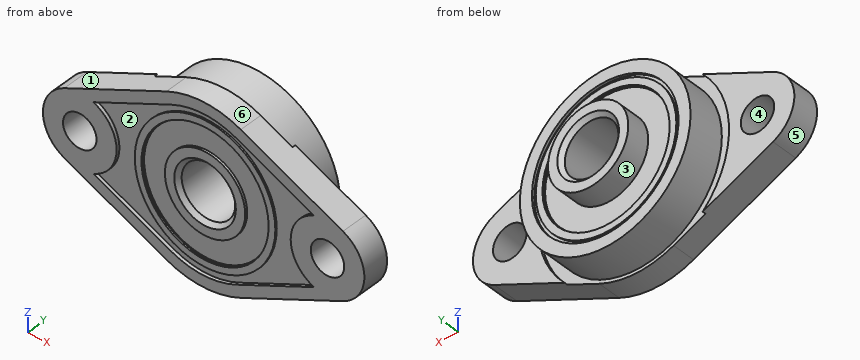
```python
from build123d import *

# Parameters (mm, degrees)
SKETCH2_R               = 2.5
BOSS_EXTRUDE1_DEPTH     = 4
SKETCH3_R               = 14.25
CUT_EXTRUDE1_DEPTH      = 0.5
SKETCH4_R               = 12.75
BOSS_EXTRUDE2_DEPTH     = 5.5
CUT_EXTRUDE2_DEPTH      = 0.5
SKETCH6_R               = 10.95
CUT_EXTRUDE3_DEPTH      = 0.4
SKETCH7_R               = 10.5
BOSS_EXTRUDE3_DEPTH     = 0.25
SKETCH8_R               = 9.5
CUT_EXTRUDE4_DEPTH      = 0.35
SKETCH9_R               = 10.5
BOSS_EXTRUDE4_DEPTH     = 0.25
SKETCH10_R              = 9.5
CUT_EXTRUDE5_DEPTH      = 0.35
SKETCH11_R              = 6
BOSS_EXTRUDE5_DEPTH     = 0.35
SKETCH12_R              = 6
BOSS_EXTRUDE6_DEPTH     = 3.5
SKETCH13_R              = 4
CUT_EXTRUDE6_DEPTH      = 1
CUT_EXTRUDE6_DEPTH_BACK = 13
CHAMFER1_SIZE           = 0.6
CHAMFER2_SIZE           = 0.6
CHAMFER3_SIZE           = 0.1


with BuildPart() as part:
    # Sketch2 → Boss-Extrude1 (new body)
    with BuildSketch(Plane(origin=(0, 0, 0), x_dir=(1, 0, 0), z_dir=(0, 1, 0))):
        with BuildLine():
            Line((-5.550675676, 12.031313293), (-20.804054054, 4.994130046))
            ThreePointArc((-20.804054054, 4.994130046), (-24, 0), (-20.804054054, -4.994130046))
            Line((-20.804054054, -4.994130046), (-5.550675676, -12.031313293))
            ThreePointArc((-5.550675676, -12.031313293), (0, -13.25), (5.550675676, -12.031313293))
            Line((5.550675676, -12.031313293), (20.804054054, -4.994130046))
            ThreePointArc((20.804054054, -4.994130046), (24, 0), (20.804054054, 4.994130046))
            Line((20.804054054, 4.994130046), (5.550675676, 12.031313293))
            ThreePointArc((5.550675676, 12.031313293), (0, 13.25), (-5.550675676, 12.031313293))
        make_face()
        with Locations((-18.5, 0)):
            Circle(SKETCH2_R, mode=Mode.SUBTRACT)
        with Locations((18.5, 0)):
            Circle(SKETCH2_R, mode=Mode.SUBTRACT)
    extrude(amount=BOSS_EXTRUDE1_DEPTH)

    # Sketch3 → Cut-Extrude1 (cut)
    with BuildSketch(Plane(origin=(0, 4, 0), x_dir=(1, 0, 0), z_dir=(0, 1, 0))):
        Circle(SKETCH3_R)
    extrude(amount=-CUT_EXTRUDE1_DEPTH, mode=Mode.SUBTRACT)

    # Sketch4 → Boss-Extrude2 (add)
    with BuildSketch(Plane(origin=(0, 3.5, 0), x_dir=(1, 0, 0), z_dir=(0, 1, 0))):
        Circle(SKETCH4_R)
    extrude(amount=BOSS_EXTRUDE2_DEPTH)

    # Sketch5 → Cut-Extrude2 (cut)
    with BuildSketch(Plane.XZ):
        with BuildLine():
            Line((4.838513514, -10.487673097), (16.48142728, -5.116186488))
            ThreePointArc((16.48142728, -5.116186488), (13, 0), (16.48142728, 5.116186488))
            Line((16.48142728, 5.116186488), (4.838513514, 10.487673097))
            ThreePointArc((4.838513514, 10.487673097), (0, 11.55), (-4.838513514, 10.487673097))
            Line((-4.838513514, 10.487673097), (-16.48142728, 5.116186488))
            ThreePointArc((-16.48142728, 5.116186488), (-13, 0), (-16.48142728, -5.116186488))
            Line((-16.48142728, -5.116186488), (-4.838513514, -10.487673097))
            ThreePointArc((-4.838513514, -10.487673097), (0, -11.55), (4.838513514, -10.487673097))
        make_face()
    extrude(amount=-CUT_EXTRUDE2_DEPTH, mode=Mode.SUBTRACT)

    # Sketch6 → Cut-Extrude3 (cut)
    with BuildSketch(Plane(origin=(0, 9, 0), x_dir=(1, 0, 0), z_dir=(0, 1, 0))):
        Circle(SKETCH6_R)
    extrude(amount=-CUT_EXTRUDE3_DEPTH, mode=Mode.SUBTRACT)

    # Sketch7 → Boss-Extrude3 (add)
    with BuildSketch(Plane(origin=(0, 8.6, 0), x_dir=(1, 0, 0), z_dir=(0, 1, 0))):
        Circle(SKETCH7_R)
    extrude(amount=BOSS_EXTRUDE3_DEPTH)

    # Sketch8 → Cut-Extrude4 (cut)
    with BuildSketch(Plane(origin=(0, 8.85, 0), x_dir=(1, 0, 0), z_dir=(0, 1, 0))):
        Circle(SKETCH8_R)
    extrude(amount=-CUT_EXTRUDE4_DEPTH, mode=Mode.SUBTRACT)

    # Sketch9 → Boss-Extrude4 (add)
    with BuildSketch(Plane.XZ.offset(-0.5)):
        Circle(SKETCH9_R)
    extrude(amount=BOSS_EXTRUDE4_DEPTH)

    # Sketch10 → Cut-Extrude5 (cut)
    with BuildSketch(Plane.XZ.offset(-0.25)):
        Circle(SKETCH10_R)
    extrude(amount=-CUT_EXTRUDE5_DEPTH, mode=Mode.SUBTRACT)

    # Sketch11 → Boss-Extrude5 (add)
    with BuildSketch(Plane.XZ.offset(-0.6)):
        Circle(SKETCH11_R)
    extrude(amount=BOSS_EXTRUDE5_DEPTH)

    # Sketch12 → Boss-Extrude6 (add)
    with BuildSketch(Plane(origin=(0, 8.5, 0), x_dir=(1, 0, 0), z_dir=(0, 1, 0))):
        Circle(SKETCH12_R)
    extrude(amount=BOSS_EXTRUDE6_DEPTH)

    # Sketch13 → Cut-Extrude6 (cut, two sides)
    with BuildSketch(Plane(origin=(0, 12, 0), x_dir=(1, 0, 0), z_dir=(0, 1, 0))) as cut_extrude6_sk:
        Circle(SKETCH13_R)
    extrude(amount=CUT_EXTRUDE6_DEPTH, mode=Mode.SUBTRACT)
    extrude(cut_extrude6_sk.sketch, amount=-CUT_EXTRUDE6_DEPTH_BACK, mode=Mode.SUBTRACT)

    # Chamfer1
    chamfer1_edges = [part.edges().sort_by_distance(p)[0] for p in [
        (-4, 12, 0),
    ]]
    chamfer(chamfer1_edges, length=CHAMFER1_SIZE)

    # Chamfer2
    chamfer2_edges = [part.edges().sort_by_distance(p)[0] for p in [
        (-4, 0.25, 0),
    ]]
    chamfer(chamfer2_edges, length=CHAMFER2_SIZE)

    # Chamfer3
    chamfer3_edges = [part.edges().sort_by_distance(p)[0] for p in [
        (-9.5, 0.6, 0),
        (-9.5, 8.5, 0),
    ]]
    chamfer(chamfer3_edges, length=CHAMFER3_SIZE)


solid = part.part
```
Read the model definition and answer for the solid it produces. Units are mm, in the model's axes. Face numbers are marked on the shaded views. A direction names the side the tool comes from. Give positions to 0.01 mm unless a question says otherwise; leave off trailing zeros. Write each loop counter-clockwise with the first axis right and the second up, starting at its lowest first coordinate (ties: lowest second). Pieces come first, ordered by that corner, then holes. Notation, with made-up numbers: (68, 40.25) - (116, 40.25) arc R16 cw to (116, 67.25) - close; hole circle Ø1 at (63, -2.75). An arc over 180 degrees is marked (long way). Write item = value, one per line. Start each with the question number.
Item 1: Each of these flat-tipped pins is pushed along its axis until it touches: P1, Ø6.5, axis at x = 0, z = -4, coming from the +Y side; P2, Ø4.5, axis at x = 18.5, z = 0, coming from the +Y side (3 decimals); P3, Ø13, axis at x = 0, z = 0, coming from the -Y side; P4, Ø1.5, axis at y = 6, z = 3.5, coming from the +X side. Where does it stop, or does it pass through?
Item 2: Find section A-A (y = 1.75). Give the vertices of the cut face in (x, z).
Item 3: A tool of negligible diameter and unlimited length cuts with its end or side. For the marked faces 1, 2 and 3, from which of +Z, -Z, +X, -X, +Y, -Y can it reach the whole face along a straight path? Write none if from no direction.
Item 4: Find the intervals of material crossed by probe 1 along X at (y, z) = (8.75, 0); probe 2 along X at (y, z) = (8.9, 0), in increasing order. Write a range as [from, to].
Item 5: Find section C-C (y = 10.75). Give the vertices of the cut face in (x, z).
Item 6: Find section D-D (z = 0). State how many separate pieces and enclosed holes the cut face has, then the cut area to 3 significant figures.
Item 7: Find section B-B (x = 19). Give the vertices of the cut face in (y, z).
Item 8: The mould has two halves that part along X. Classify the marked faces 4, 5 and 6: +X half, -X half, draft (parallel to the pull), parting line (faces both ways), or undercut.
Response:
q1.P1 = 12
q1.P2 = through
q1.P3 = 0.25
q1.P4 = 12.45
q2.outline = (-20.8, -4.99) - (-5.55, -12.03) arc R13.25 ccw to (5.55, -12.03) - (20.8, -4.99) arc R5.5 ccw to (20.8, 4.99) - (5.55, 12.03) arc R13.25 ccw to (-5.55, 12.03) - (-20.8, 4.99) arc R5.5 ccw to start; hole circle Ø5 at (-18.5, 0); hole circle Ø8 at (0, 0); hole circle Ø5 at (18.5, 0)
q3.face_1 = +Z, -X, +Y, -Y
q3.face_2 = -Y
q3.face_3 = +Y
q4.probe_1 = [-12.75, -10.95], [-10.5, -9.5], [-6, -4], [4, 6], [9.5, 10.5], [10.95, 12.75]
q4.probe_2 = [-12.75, -10.95], [-6, -4], [4, 6], [10.95, 12.75]
q5.outline = circle Ø12 at (0, 0); hole circle Ø8 at (0, 0)
q6.separate_pieces = 4
q6.enclosed_holes = 0
q6.area = 205 mm²
q7.outline = (0, -5.83) - (4, -5.83) - (4, -2.45) - (0, -2.45) - close; (0, 2.45) - (4, 2.45) - (4, 5.83) - (0, 5.83) - close
q8.face_4 = undercut
q8.face_5 = -X half
q8.face_6 = parting line
